For this review, take the finished solid that the model builds, in its own axes (mm). Face numbers are marked on the shaded views. A direction names the side the tool comes from. Round coordinates to 2 decimals unless told otherwise and drop trailing zeros. Loops run counter-clockwise (first coordinate to the right, second up) from the corner with the lowest first, then second, coordinate; pieces in that order, holes last. Notation, with made-up numbers: (87, 73) -> (91, 73) arc R21 cw to (91, 108) -> close; hole circle Ø2 at (-23, 7.25). An arc over 180 degrees is marked (long way). One line per question, with ' | ' between items. Start each with the question number.
1. Consider section D-D (z = 6). Write out the cut boundary in (x, y).
2. Consider section B-B (z = 11.75). Write out the cut boundary in (x, y), and give its area (3 significant figures).
3. Consider section A-A (x = 0). Write out the cut boundary in (y, z), and give its area (3 significant figures).
4. For pin 1 Ø3 at (x, y) = (2, 4) entering from +Z; pin 2 Ø9.5 at (x, y) = (2.5, 8) entering from +Z; pin 3 Ø6 at (y, z) = (12, 8.5) entering from +X; pin 4 Ø4 at (y, z) = (6, 9) entering from +X, all flat-tipped, find the tip position at first contact; note any pin that passes through.
5. Draft analysis for pull direction Y (two halves, no side actions). For the marked faces 3, 4 and 5, state which applies: pulls with the +Y half, pulls with the -Y half, needs draft (parallel to the pull), parting line crosses it, or undercut.
6. For the marked faces 1 and 2, list the 3-axis set-ups (+Z, -Z, +X, -X, +Y, -Y) from which the entire face can be reached by the end or side of a thin tool; tool diameter is ignored.
7. Wall thickness on line 1 along Y through (x, z) = (0, 12.6); line 2 along X through (y, z) = (4, 14.25); line 3 along Y through (x, z) = (11, 13.75): over which ranges is each line inside the solid? List them lowest first.
```python
from build123d import *

# Parameters (mm, degrees)
SKETCH1_R           = 20
BOSS_EXTRUDE1_DEPTH = 15
SKETCH2_R           = 10
CUT_EXTRUDE1_DEPTH  = 5
SKETCH3_R           = 16.129464202
SKETCH3_R_2         = 14.05591846
CUT_EXTRUDE2_DEPTH  = 8


with BuildPart() as part:
    # Sketch1 → Boss-Extrude1 (new body)
    with BuildSketch(Plane.XY):
        Circle(SKETCH1_R)
    extrude(amount=BOSS_EXTRUDE1_DEPTH)

    # Sketch2 → Cut-Extrude1 (cut)
    with BuildSketch(Plane.XY.offset(15)):
        Circle(SKETCH2_R)
    extrude(amount=-CUT_EXTRUDE1_DEPTH, mode=Mode.SUBTRACT)

    # Sketch3 → Cut-Extrude2 (cut)
    with BuildSketch(Plane.XY.offset(15)):
        Circle(SKETCH3_R)
        Circle(SKETCH3_R_2, mode=Mode.SUBTRACT)
    extrude(amount=-CUT_EXTRUDE2_DEPTH, mode=Mode.SUBTRACT)


solid = part.part
```
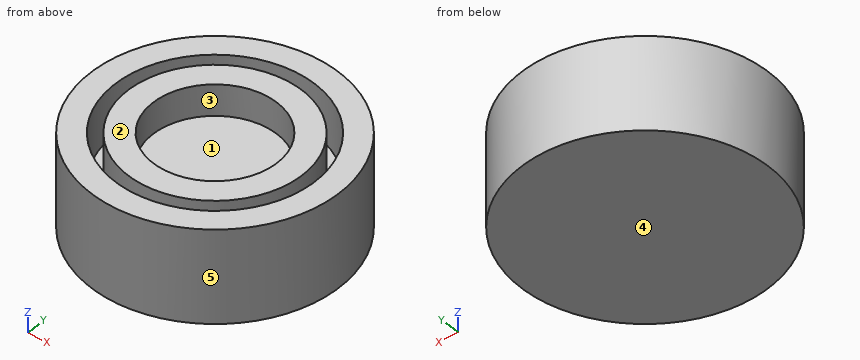
Answer block:
1) outline: circle Ø40 at (0, 0)
2) outline: circle Ø40 at (0, 0); circle Ø28.11 at (0, 0); hole circle Ø32.26 at (0, 0); hole circle Ø20 at (0, 0) | area: 746 mm2
3) outline: (-20, 0) -> (20, 0) -> (20, 15) -> (16.13, 15) -> (16.13, 7) -> (14.06, 7) -> (14.06, 15) -> (10, 15) -> (10, 10) -> (-10, 10) -> (-10, 15) -> (-14.06, 15) -> (-14.06, 7) -> (-16.13, 7) -> (-16.13, 15) -> (-20, 15) -> close | area: 467 mm2
4) pin 1: stops at z = 10 | pin 2: stops at z = 15 | pin 3: stops at x = 17.86 | pin 4: stops at x = 19.6
5) face 3: undercut | face 4: needs draft | face 5: parting line crosses it
6) face 1: +Z | face 2: +Z, +X, -X, +Y, -Y
7) line 1: y = -20 to -16.13, -14.06 to -10, 10 to 14.06, 16.13 to 20 | line 2: x = -19.6 to -15.63, -13.47 to -9.17, 9.17 to 13.47, 15.63 to 19.6 | line 3: y = -16.7 to -11.8, -8.75 to 8.75, 11.8 to 16.7
